Source: CAD feature listing. Evaluate the final solid. Frame: model axes, mm. Give positions to 0.01 mm unless a question says otherwise; leave off trailing zeros. Loops run counter-clockwise (first coordinate to the right, second up) from the corner with the lowest first, then second, coordinate; pieces in that order, holes last. Notation, with made-up numbers: (-40, 81) -> (-32, 81) arc R26 ccw to (-32, 98) -> close; hole circle Ø5 at (16, -25). An arc over 180 degrees is marked (long way). Put each result on its own line as item: value.
Autodesk Inventor part; units mm, degrees
ref_plane "YZ Plane" through (0, 0, 0) normal (1, 0, 0) x (0, 1, 0)
ref_plane "XZ Plane" through (0, 0, 0) normal (0, 1, 0) x (-1, 0, 0)
ref_plane "XY Plane" through (0, 0, 0) normal (0, 0, 1) x (1, 0, 0)
sketch "Sketch1" plane through (0, 0, 0) normal (1, 0, 0) x (0, 1, 0)
  circle A0 centre (0, 0) radius 27.94
  dimension "d0" = 55.88
extrude "Extrusion1" add sketch "Sketch1" along normal blind 5.08
sketch "Sketch3" plane through (5.08, 0, 0) normal (1, 0, 0) x (0, 0, -1)
  point P0 (0, 0)
  point P1 (15.875, 0)
  dimension "d6" = 15.875
hole "Hole1" at (5.08, 0, -15.875) direction (-1, 0, 0) diameter 3.5052 end through all
pattern_circular "Circular Pattern1" count 6 over 360 about axis through (-10, 0, 0) along (1, 0, 0) of "Hole1"
chamfer "Chamfer1" distance 2.032 angle 18 1 edges at (0, -27.94, 0) measured on face at (0, 4.0768, 2.3537)
sketch "Sketch4" plane through (5.08, 0, 0) normal (1, 0, 0) x (0, 0, -1)
  circle A0 centre (0, 0) radius 10.16
  dimension "d20" = 20.32
extrude "Extrusion3" cut sketch "Sketch4" against normal through all
chamfer "Chamfer2" distance 2.032 angle 18 1 edges at (5.08, -27.94, 0) measured on face at (5.08, -19.1807, 0)
properties part number "CHA_005_DrivePulleyCenterFlange" material "ABS Plastic"
(1) First-contact query: P1, Ø2, axis at x = 3, z = -6, coming from the -Y side; P2, Ø3, axis at y = 0, z = -15.875, coming from the -X side; P3, Ø2, axis at x = 1, z = 20.5, coming from the +Y side. Flat tips, straight axial feed; report the tip coordinate or a pass-through.
Calculated:
P1: stops at y = -27.49
P2: passes through
P3: stops at y = 20.01
(2) Draft query along Y for faces 1 (the flat face through (5.08, 11, 0)), 2 (the cylindrical face through (2.51, -3.64, -27.7)), 3 (the cylindrical face through (2.504, 0.077, 14.124)). Return one class per face: released by +Y, released by -Y, zero draft, split by the parting line, or undercut.
Calculated:
face 1: zero draft
face 2: split by the parting line
face 3: undercut
(3) Section B-B on z = 0. Return loops of the section in (x, y).
Calculated:
outline: (0, -25.91) -> (0.66, -27.94) -> (4.42, -27.94) -> (5.08, -25.91) -> (5.08, -10.16) -> (0, -10.16) -> close; (0, 10.16) -> (5.08, 10.16) -> (5.08, 25.91) -> (4.42, 27.94) -> (0.66, 27.94) -> (0, 25.91) -> close
(4) Section A-A on y = 0. Return loops of the section in (x, z).
Calculated:
outline: (0, -25.91) -> (0.66, -27.94) -> (4.42, -27.94) -> (5.08, -25.91) -> (5.08, -17.63) -> (0, -17.63) -> close; (0, -14.12) -> (5.08, -14.12) -> (5.08, -10.16) -> (0, -10.16) -> close; (0, 10.16) -> (5.08, 10.16) -> (5.08, 14.12) -> (0, 14.12) -> close; (0, 17.63) -> (5.08, 17.63) -> (5.08, 25.91) -> (4.42, 27.94) -> (0.66, 27.94) -> (0, 25.91) -> close
(5) Section C-C on x = 2.25. Return loops of the section in (y, z) (1 decimal).
Calculated:
outline: circle Ø55.9 at (0, 0); hole circle Ø3.5 at (-13.7, -7.9); hole circle Ø3.5 at (-13.7, 7.9); hole circle Ø20.3 at (0, 0); hole circle Ø3.5 at (0, -15.9); hole circle Ø3.5 at (0, 15.9); hole circle Ø3.5 at (13.7, -7.9); hole circle Ø3.5 at (13.7, 7.9)
(6) Section D-D on y = 13. Give the number of separate pieces and of enclosed holes in the cut face, then the cut area to 3 significant figures.
Calculated:
separate pieces: 3
enclosed holes: 0
area: 216 mm²
(7) Line query: probe 1 along Y at (x, z) = (2.7, -9); probe 2 along Y at (x, z) = (3.6, -7); probe 3 along Y at (x, z) = (3.75, -2). Output: solid intervals per line, ascending. Write a range as from..to.
Calculated:
probe 1: y = -26.45..-15.14, -12.35..-4.71, 4.71..12.35, 15.14..26.45
probe 2: y = -27.05..-15.23, -12.27..-7.36, 7.36..12.27, 15.23..27.05
probe 3: y = -27.87..-9.96, 9.96..27.87
